Part model, mm, in its own coordinate system. A direction names the side the tool comes from. Give positions to 0.01 mm unless a question says otherwise; leave off trailing zeros. Write each loop counter-clockwise with the first axis right and the second up, starting at its lowest first coordinate (ties: lowest second). Pieces come first, ordered by that corner, then holes. Notation, with made-up numbers: M 57,23.5 L 115,23.5 A21 cw 115,39.5 Z; hole C 22,-35.75 d4. An arc over 180 degrees is marked long. Use a Markdown table: item, result.
```python
from build123d import *

# Parameters (mm, degrees)
SKETCH1_W           = 40
SKETCH1_H           = 44
BOSS_EXTRUDE1_DEPTH = 2
SKETCH2_W           = 40
SKETCH2_H           = 2
BOSS_EXTRUDE2_DEPTH = 10
SKETCH3_W           = 15
SKETCH3_H           = 3
CUT_EXTRUDE2_DEPTH  = 45
CUT_EXTRUDE3_REACH  = 4
SKETCH4_R           = 1.017178614
SKETCH4_R_2         = 1.056475415
CUT_EXTRUDE4_REACH  = 46
SKETCH5_R           = 1
CUT_EXTRUDE5_REACH  = 14
SKETCH6_R           = 1.5


with BuildPart() as part:
    # Sketch1 → Boss-Extrude1 (new body)
    with BuildSketch(Plane(origin=(0, 0, 0), x_dir=(1, 0, 0), z_dir=(0, 1, 0))):
        with Locations((20, 22)):
            Rectangle(SKETCH1_W, SKETCH1_H)
    extrude(amount=BOSS_EXTRUDE1_DEPTH)

    # Sketch2 → Boss-Extrude2 (add)
    with BuildSketch(Plane(origin=(0, 2, 0), x_dir=(1, 0, 0), z_dir=(0, 1, 0))):
        with Locations((20, 43)):
            Rectangle(SKETCH2_W, SKETCH2_H)
        with Locations((20, 1)):
            Rectangle(SKETCH2_W, SKETCH2_H)
    extrude(amount=BOSS_EXTRUDE2_DEPTH)

    # Sketch3 → Cut-Extrude2 (cut, through all)
    with BuildSketch(Plane(origin=(0, 0, -44), x_dir=(-1, 0, 0), z_dir=(0, 0, -1))):
        with Locations((-7.5, 10.5)):
            Rectangle(SKETCH3_W, SKETCH3_H)
    extrude(amount=-CUT_EXTRUDE2_DEPTH, mode=Mode.SUBTRACT)

    # Sketch4 → Cut-Extrude3 (cut, up to next)
    with BuildSketch(Plane(origin=(0, 0, -42), x_dir=(-1, 0, 0), z_dir=(0, 0, -1)), mode=Mode.PRIVATE) as cut_extrude3_sk1:
        with Locations((-35, 7)):
            Circle(SKETCH4_R)
    cut_extrude3_tool1 = extrude(cut_extrude3_sk1.sketch, amount=CUT_EXTRUDE3_REACH, mode=Mode.PRIVATE) & part.part
    add(cut_extrude3_tool1.solids().sort_by_distance((35, 7, -42))[0], mode=Mode.SUBTRACT)
    # Sketch4 → Cut-Extrude3 (cut, up to next)
    with BuildSketch(Plane(origin=(0, 0, -42), x_dir=(-1, 0, 0), z_dir=(0, 0, -1)), mode=Mode.PRIVATE) as cut_extrude3_sk2:
        with Locations((-19, 7)):
            Circle(SKETCH4_R_2)
    cut_extrude3_tool2 = extrude(cut_extrude3_sk2.sketch, amount=CUT_EXTRUDE3_REACH, mode=Mode.PRIVATE) & part.part
    add(cut_extrude3_tool2.solids().sort_by_distance((19, 7, -42))[0], mode=Mode.SUBTRACT)

    # Sketch5 → Cut-Extrude4 (cut, up to next)
    with BuildSketch(Plane.XY, mode=Mode.PRIVATE) as cut_extrude4_sk1:
        with Locations((27, 8.5)):
            Circle(SKETCH5_R)
    cut_extrude4_tool1 = extrude(cut_extrude4_sk1.sketch, amount=-CUT_EXTRUDE4_REACH, mode=Mode.PRIVATE) & part.part
    add(cut_extrude4_tool1.solids().sort_by_distance((27, 8.5, 0))[0], mode=Mode.SUBTRACT)

    # Sketch6 → Cut-Extrude5 (cut, up to next)
    with BuildSketch(Plane.XZ, mode=Mode.PRIVATE) as cut_extrude5_sk1:
        with Locations((10.909090909, -32)):
            Circle(SKETCH6_R)
    cut_extrude5_tool1 = extrude(cut_extrude5_sk1.sketch, amount=-CUT_EXTRUDE5_REACH, mode=Mode.PRIVATE) & part.part
    add(cut_extrude5_tool1.solids().sort_by_distance((10.909091, 0, -32))[0], mode=Mode.SUBTRACT)
    # Sketch6 → Cut-Extrude5 (cut, up to next)
    with BuildSketch(Plane.XZ, mode=Mode.PRIVATE) as cut_extrude5_sk2:
        with Locations((10.909090909, -12)):
            Circle(SKETCH6_R)
    cut_extrude5_tool2 = extrude(cut_extrude5_sk2.sketch, amount=-CUT_EXTRUDE5_REACH, mode=Mode.PRIVATE) & part.part
    add(cut_extrude5_tool2.solids().sort_by_distance((10.909091, 0, -12))[0], mode=Mode.SUBTRACT)
    # Sketch6 → Cut-Extrude5 (cut, up to next)
    with BuildSketch(Plane.XZ, mode=Mode.PRIVATE) as cut_extrude5_sk3:
        with Locations((30.909090909, -12)):
            Circle(SKETCH6_R)
    cut_extrude5_tool3 = extrude(cut_extrude5_sk3.sketch, amount=-CUT_EXTRUDE5_REACH, mode=Mode.PRIVATE) & part.part
    add(cut_extrude5_tool3.solids().sort_by_distance((30.909091, 0, -12))[0], mode=Mode.SUBTRACT)
    # Sketch6 → Cut-Extrude5 (cut, up to next)
    with BuildSketch(Plane.XZ, mode=Mode.PRIVATE) as cut_extrude5_sk4:
        with Locations((30.909090909, -32)):
            Circle(SKETCH6_R)
    cut_extrude5_tool4 = extrude(cut_extrude5_sk4.sketch, amount=-CUT_EXTRUDE5_REACH, mode=Mode.PRIVATE) & part.part
    add(cut_extrude5_tool4.solids().sort_by_distance((30.909091, 0, -32))[0], mode=Mode.SUBTRACT)


solid = part.part
```
1. Cut at D-D, the plane y = 1.5. Give the cut face in (x, z).
Findings below:
| item | result |
|---|---|
| outline | M 0,-44 L 40,-44 L 40,0 L 0,0 Z; hole C 10.91,-32 d3; hole C 10.91,-12 d3; hole C 30.91,-32 d3; hole C 30.91,-12 d3 |
2. Two-plate mould, pull along Y, no slides. Class faces 4 (the cylindrical face through (18.024, 6.595, -42.986)), 5 (the cylindrical face through (29.41, 0.99, -31.93)), 6 (the flat face through (27, 12, -43)): released by +Y, released by -Y, zero draft, split by the parting line, or undercut.
Findings below:
| item | result |
|---|---|
| face 4 | undercut |
| face 5 | zero draft |
| face 6 | released by +Y |
3. Drill centre lines: L1, parallel to X at y = 7, z = -43.5; L2, parallel to Z at x = 11, y = 8.75; L3, parallel to Y at x = 35, z = -42.5. Where is each one in solid material? Low to high.
Findings below:
| item | result |
|---|---|
| L1 | 0 to 17.94, 20.06 to 33.98, 36.02 to 40 |
| L2 | -44 to -42, -2 to 0 |
| L3 | 0 to 5.98, 8.02 to 12 |
4. Cut at B-B, the plane x = 19. Give the cut face in (y, z), then the cut area to 3 significant figures.
Findings below:
| item | result |
|---|---|
| outline | M 0,-44 L 5.94,-44 L 5.94,-42 L 2,-42 L 2,-2 L 12,-2 L 12,0 L 0,0 Z; M 8.06,-44 L 12,-44 L 12,-42 L 8.06,-42 Z |
| area | 124 mm2 |
5. Tool access for faces 1 (the flat face through (20, 2, -22)), 2 (the cylindrical face through (26.87, 9.49, -0.99)), 3 (the flat face through (15, 10, -43)): list every direction of +Z, -Z, +X, -X, +Y, -Y with a clear straight run to the whole face (end or side of a thin tool).
Findings below:
| item | result |
|---|---|
| face 1 | +X, -X, +Y |
| face 2 | +Z |
| face 3 | +Z, -Z, -X, +Y |
6. Drop flat-ended pins along their axis: P1, Ø2.5, axis at x = 19, y = 7, coming from the +Z side; P2, Ø1.6, axis at y = 10.5, z = -43, coming from the -X side; P3, Ø20, axis at x = 28, z = -17.5, coming from the +Y side; P4, Ø1, axis at x = 11, z = -43.5, coming from the +Y side. Give the stop position or say it passes through.
Findings below:
| item | result |
|---|---|
| P1 | z = 0 |
| P2 | x = 15 |
| P3 | y = 2 |
| P4 | y = 9 |
7. Cut at A-A, the plane y = 7. Give the cut face in (x, z).
Findings below:
| item | result |
|---|---|
| outline | M 0,-44 L 17.94,-44 L 17.94,-42 L 0,-42 Z; M 0,-2 L 40,-2 L 40,0 L 0,0 Z; M 20.06,-44 L 33.98,-44 L 33.98,-42 L 20.06,-42 Z; M 36.02,-44 L 40,-44 L 40,-42 L 36.02,-42 Z |
8. Cut at C-C, the plane z = -12. Give the cut face in (x, y).
Findings below:
| item | result |
|---|---|
| outline | M 0,0 L 9.41,0 L 9.41,2 L 0,2 Z; M 12.41,0 L 29.41,0 L 29.41,2 L 12.41,2 Z; M 32.41,0 L 40,0 L 40,2 L 32.41,2 Z |
